```python
from build123d import *

# Parameters (mm, degrees)
SALIENTE_EXTRUIR1_DEPTH = 20
SALIENTE_EXTRUIR2_DEPTH = 20
CROQUIS3_W              = 30
CROQUIS3_H              = 4
CORTAR_EXTRUIR1_DEPTH   = 4


with BuildPart() as part:
    # Croquis1 → Saliente-Extruir1 (new body)
    with BuildSketch(Plane.XY):
        with BuildLine():
            Line((-28, 0), (-25, 0))
            ThreePointArc((-25, 0), (0, 25), (25, 0))
            Line((25, 0), (28, 0))
            ThreePointArc((28, 0), (0, 28), (-28, 0))
        make_face()
    extrude(amount=SALIENTE_EXTRUIR1_DEPTH)

    # Croquis2 → Saliente-Extruir2 (add)
    with BuildSketch(Plane.XY.offset(20)):
        Polygon((0, 28), (15, 28), (15, 22.565689598), (0, 26.315842258), (-15, 21.969074402), (-15, 28), align=None)
    extrude(amount=-SALIENTE_EXTRUIR2_DEPTH)

    # Croquis3 → Cortar-Extruir1 (cut)
    with BuildSketch(Plane(origin=(0, 28, 0), x_dir=(1, 0, 0), z_dir=(0, 1, 0))):
        with Locations((0, -15)):
            Rectangle(CROQUIS3_W, CROQUIS3_H)
        with Locations((0, -5)):
            Rectangle(CROQUIS3_W, CROQUIS3_H)
    extrude(amount=-CORTAR_EXTRUIR1_DEPTH, mode=Mode.SUBTRACT)


solid = part.part
```
Geometry check sheet. Reference: the model listing, model coordinates, mm. A direction names the side the tool comes from. Coordinates: 2 decimals unless noted, no trailing zeros. Order: outer loops, then holes, each group sorted by start corner. A loop starts at its lowest first (then second) coordinate and runs counter-clockwise, first axis right, second up.
Q1. Sectioned sample at B-B on x = 0. Record the cut outline in (y, z), and give its area (3 significant figures).
Reply:
outline: (25, 0) - (28, 0) - (28, 3) - (25, 3) - close; (25, 7) - (28, 7) - (28, 13) - (25, 13) - close; (25, 17) - (28, 17) - (28, 20) - (25, 20) - close
area: 36.0 mm2
Q2. Sectioned sample at C-C on z = 6. Record the cut outline in (x, y), and give its area (3 significant figures).
Reply:
outline: (-28, 0) - (-25, 0) arc R25 cw to (-7, 24) - (-15, 24) - (-15, 23.64) arc R28 ccw to start; (7, 24) arc R25 cw to (25, 0) - (28, 0) arc R28 ccw to (15, 23.64) - (15, 24) - close
area: 181 mm2
Q3. Depth check by flat-ended pin: pin 1 Ø2 at (y, z) = (20, 2.5) entering from -X; pin 2 Ø2 at (x, z) = (-10.5, 15.5) entering from +Y; pin 3 Ø4 at (x, z) = (7, 4) entering from -Y. Enter the tip coordinate at first touch or a pass-through.
Reply:
pin 1: stops at x = -20.57
pin 2: stops at y = 24
pin 3: stops at y = 23.32
Q4. Tool access check on faces 1 (the face through (0, 26, 7)), 2 (the face through (-15, 26, 10)), 3 (the face through (15, 26, 10)), 4 (the face through (0, 28, 19)). Record the directions out of +Z, -Z, +X, -X, +Y, -Y that give a thin tool (end or side, any length) a straight path to the whole face; none if there is none.
Reply:
face 1: +X, -X, +Y
face 2: +Z, -Z, -X, +Y
face 3: +Z, -Z, +X, +Y
face 4: +Z, -Z, +X, -X, +Y
Q5. Sectioned sample at D-D on y = 5.5. Record the cut outline in (x, z).
Reply:
outline: (-27.45, 0) - (-24.39, 0) - (-24.39, 20) - (-27.45, 20) - close; (24.39, 0) - (27.45, 0) - (27.45, 20) - (24.39, 20) - close
Q6. Sectioned sample at A-A on y = 26.25. Record the cut outline in (x, z), and give its area (3 significant figures).
Reply:
outline: (-15, 0) - (15, 0) - (15, 3) - (-15, 3) - close; (-15, 7) - (15, 7) - (15, 13) - (-15, 13) - close; (-15, 17) - (15, 17) - (15, 20) - (-15, 20) - close
area: 360 mm2
Q7. Thickness scan on probe 1 along Z at (x, y) = (9, 25.25); probe 2 along X at (y, z) = (17.5, 7.75); probe 3 along X at (y, z) = (3, 7.75). Record the ranges inside material, lowest first.
Reply:
probe 1: z = 0 to 3, 7 to 13, 17 to 20
probe 2: x = -21.86 to -17.85, 17.85 to 21.86
probe 3: x = -27.84 to -24.82, 24.82 to 27.84
